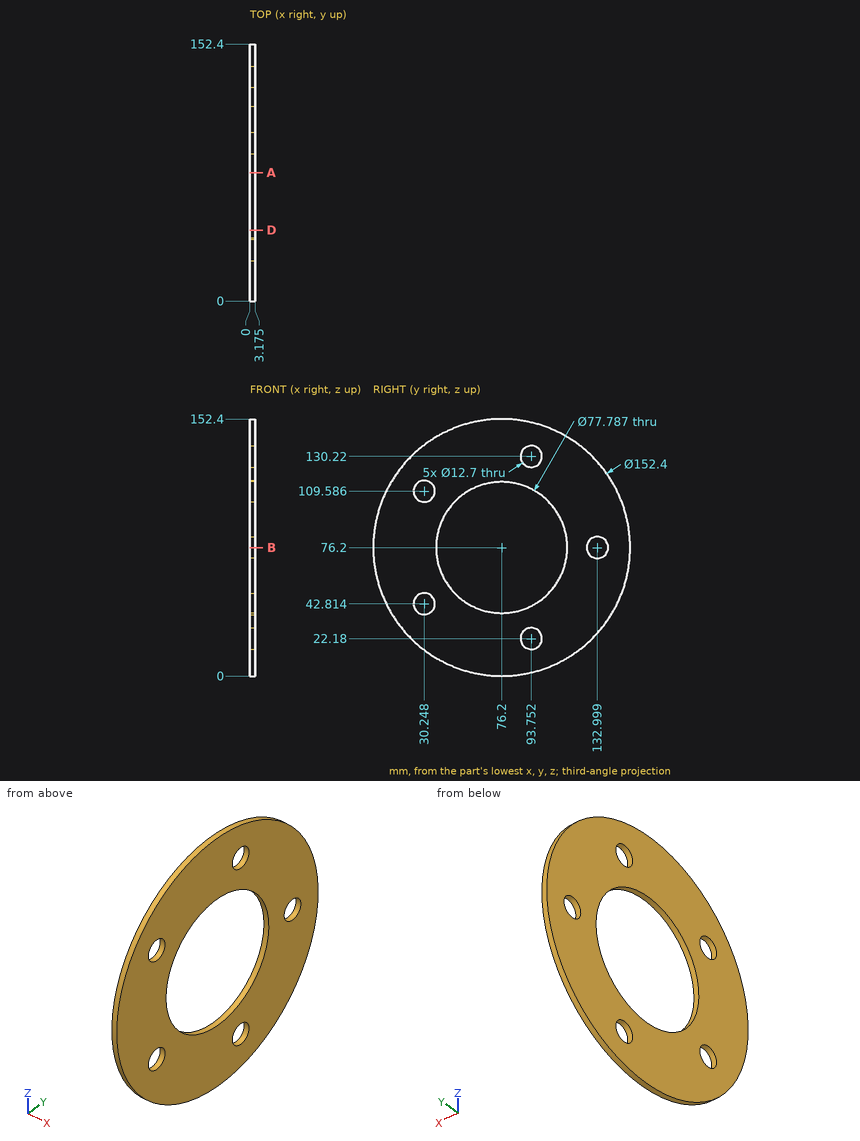
Geometry check sheet. Reference: drawing and pictorial views, mm from the part's lowest x, y, z. Coordinates: 2 decimals unless noted, no trailing zeros. Order: outer loops, then holes, each group sorted by start corner. A loop starts at its lowest first (then second) coordinate and runs counter-clockwise, first axis right, second up. Notation, with made-up numbers: M 32,-28.5 L 74,-28.5 A22 ccw 74,10.5 Z; hole C 16.25,2 d8. An arc over 180 degrees is marked long. Return JSON: item names as keys, results as strings.
1) Cross-section at B-B, the plane z = 76.2. Count the separate pieces of the cut face and the enclosed holes in it.
Answer list:
{"separate pieces": "3", "enclosed holes": "0"}
2) Thickness scan on L1, parallel to Y at x = 2.2, z = 76.2; L2, parallel to Z at x = 0.5, y = 92 (1 decimal); L3, parallel to Y at x = 1.25, z = 108.5 (1 decimal). Record the ranges inside material, lowest first. Write a range as [from, to].
Answer list:
{"L1": "[0, 37.31], [115.09, 126.65], [139.35, 152.4]", "L2": "[1.7, 16.1], [28.3, 40.7], [111.7, 124.1], [136.3, 150.7]", "L3": "[7.2, 24], [36.5, 54.5], [97.9, 145.2]"}
3) Gauge pin test, flat ends, axial feed: pin 1 (11.5 mm diameter, centred on y = 133, z = 76.2, fed in from -X); pin 2 (1 mm diameter, centred on x = 2, z = 48.5, fed in from -Y); pin 3 (1.5 mm diameter, centred on x = 1.5, y = 109.5, fed in from -Z). Record the tip position at first contact, or that the pin passes through.
Answer list:
{"pin 1": "through", "pin 2": "y = 5.02", "pin 3": "z = 7.3"}
4) Cross-section at A-A, the plane y = 76.2. Record the boundary of the cut face in (x, z) (1 decimal).
Answer list:
{"outline": "M 0,0 L 3.2,0 L 3.2,37.3 L 0,37.3 Z; M 0,115.1 L 3.2,115.1 L 3.2,152.4 L 0,152.4 Z"}
5) Cross-section at D-D, the plane y = 42. Record the boundary of the cut face in (x, z) (1 decimal), and give its area (3 significant figures).
Answer list:
{"outline": "M 0,8.1 L 3.2,8.1 L 3.2,57.7 L 0,57.7 Z; M 0,94.7 L 3.2,94.7 L 3.2,144.3 L 0,144.3 Z", "area": "315 mm2"}
